from build123d import *

# Parameters (mm, degrees)
F1_DEPTH     = 20
F2_DEPTH     = 5
F3_R         = 6.25
F4_DEPTH     = 10
F5_R         = 1.4
F6_DEPTH     = 3.9098179487
F7_T1_DEPTH  = 47.5
F7_T3_DEPTH  = 32.5
F7_T5_DEPTH  = 20.5
F7_T7_DEPTH  = 35.5
F7_T9_DEPTH  = 10
F7_S13_W     = 5
F7_S13_H     = 5
F7_T14_DEPTH = 5
F7_S19_W     = 5
F7_S19_H     = 5
F7_T20_DEPTH = 5
F7_T27_DEPTH = 45
F7_T31_DEPTH = 33
F7_T38_DEPTH = 45
F7_T42_DEPTH = 33


# Not quite as in the source:
# - a fillet or chamfer that OpenCascade refuses, or shapes differently, is made with other operations: its cross-section is extruded or revolved along the edge and cut away or added


with BuildPart() as f1:
    # F0 (on Top) → F1 (new body)
    with BuildSketch(Plane.XY):
        Polygon((0, 10), (0, 0), (0, -10), (20, -10), (20, -18), (40, -18), (40, 10), align=None)
        Polygon((35.5, -12), (35.5, -17.5), (30, -17.5), (24.5, -17.5), (24.5, -12), align=None, mode=Mode.SUBTRACT)
    extrude(amount=F1_DEPTH)

    # F0 (on Top) → F2 (join)
    with BuildSketch(Plane.XY):
        Polygon((30, -17.5), (35.5, -17.5), (35.5, -12), (24.5, -12), (24.5, -17.5), align=None)
    extrude(amount=F2_DEPTH)

    # F3 (on face) → F4 (cut)
    with BuildSketch(Plane(origin=(0, 0, 0), x_dir=(0, -1, 0), z_dir=(-1, 0, 0))):
        with Locations((0, 10)):
            Circle(F3_R)
    extrude(amount=-F4_DEPTH, mode=Mode.SUBTRACT)

    # F5 (on face) → F6 (cut, through all)
    with BuildSketch(Plane(origin=(0, 10, 0), x_dir=(-1, 0, 0), z_dir=(0, 1, 0))):
        with Locations((-5, 10)):
            Circle(F5_R)
    extrude(amount=-F6_DEPTH, mode=Mode.SUBTRACT)

    # F7: fillet of radius 5 on 9 edges, made by hand

    # F7_s2 → F7_t1 (cut)
    with BuildSketch(Plane.YZ.offset(-12.5)):
        with BuildLine():
            ThreePointArc((10, 15), (8.5355339059, 18.5355339059), (5, 20))
            Line((5, 20), (10, 20))
            Line((10, 20), (10, 15))
        make_face()
        with BuildLine():
            ThreePointArc((10, 5), (8.5355339059, 1.4644660941), (5, 0))
            Line((5, 0), (10, 0))
            Line((10, 0), (10, 5))
        make_face()
    extrude(amount=F7_T1_DEPTH, mode=Mode.SUBTRACT)

    # F7_s4 → F7_t3 (cut)
    with BuildSketch(Plane.YZ.offset(-12.5)):
        with BuildLine():
            ThreePointArc((-5, 20), (-8.5355339059, 18.5355339059), (-10, 15))
            Line((-10, 15), (-10, 20))
            Line((-10, 20), (-5, 20))
        make_face()
        with BuildLine():
            ThreePointArc((-5, 0), (-8.5355339059, 1.4644660941), (-10, 5))
            Line((-10, 5), (-10, 0))
            Line((-10, 0), (-5, 0))
        make_face()
    extrude(amount=F7_T3_DEPTH, mode=Mode.SUBTRACT)

    # F7_s6 → F7_t5 (cut)
    with BuildSketch(Plane.XZ.offset(10)):
        with BuildLine():
            ThreePointArc((25, 20), (21.4644660941, 18.5355339059), (20, 15))
            Line((20, 15), (20, 20))
            Line((20, 20), (25, 20))
        make_face()
        with BuildLine():
            ThreePointArc((25, 0), (21.4644660941, 1.4644660941), (20, 5))
            Line((20, 5), (20, 0))
            Line((20, 0), (25, 0))
        make_face()
    extrude(amount=F7_T5_DEPTH, mode=Mode.SUBTRACT)

    # F7_s8 → F7_t7 (cut)
    with BuildSketch(Plane.XZ.offset(-5)):
        with BuildLine():
            ThreePointArc((35, 20), (38.5355339059, 18.5355339059), (40, 15))
            Line((40, 15), (40, 20))
            Line((40, 20), (35, 20))
        make_face()
        with BuildLine():
            ThreePointArc((35, 0), (38.5355339059, 1.4644660941), (40, 5))
            Line((40, 5), (40, 0))
            Line((40, 0), (35, 0))
        make_face()
    extrude(amount=F7_T7_DEPTH, mode=Mode.SUBTRACT)

    # F7_s10 → F7_t9 (cut)
    with BuildSketch(Plane.XY.offset(5)):
        with BuildLine():
            ThreePointArc((35, 10), (38.5355339059, 8.5355339059), (40, 5))
            Line((40, 5), (40, 10))
            Line((40, 10), (35, 10))
        make_face()
    extrude(amount=F7_T9_DEPTH, mode=Mode.SUBTRACT)


with BuildPart() as f7_tool12:
    # F7_s13 → F7_t14 (new body)
    with BuildSketch(Plane.XZ.offset(-5)):
        with Locations((37.5, 17.5)):
            Rectangle(F7_S13_W, F7_S13_H)
    extrude(amount=-F7_T14_DEPTH)

    # F7_s15 → F7_t16 (revolve, cut)
    with BuildSketch(Plane(origin=(35, 5, 15), x_dir=(-0.7071067812, 0, -0.7071067812), z_dir=(0.7071067812, 0, -0.7071067812))):
        with BuildLine():
            ThreePointArc((0, -5), (5, 0), (0, 5))
            Line((0, 5), (0, -5))
        make_face()
    revolve(axis=Axis((35, 5, 15), (0, 1, 0)), mode=Mode.SUBTRACT)


with BuildPart() as f1_1:
    add(f1.part)

    # F7_t11: cut F7_tool12
    add(f7_tool12.part, mode=Mode.SUBTRACT)


with BuildPart() as f7_tool18:
    # F7_s19 → F7_t20 (new body)
    with BuildSketch(Plane.XZ.offset(-5)):
        with Locations((37.5, 2.5)):
            Rectangle(F7_S19_W, F7_S19_H)
    extrude(amount=-F7_T20_DEPTH)

    # F7_s21 → F7_t22 (revolve, cut)
    with BuildSketch(Plane(origin=(35, 5, 5), x_dir=(-0.7071067812, 0, 0.7071067812), z_dir=(-0.7071067812, 0, -0.7071067812))):
        with BuildLine():
            ThreePointArc((0, -5), (5, 0), (0, 5))
            Line((0, 5), (0, -5))
        make_face()
    revolve(axis=Axis((35, 5, 5), (0, 1, 0)), mode=Mode.SUBTRACT)


with BuildPart() as f1_2:
    add(f1_1.part)

    # F7_t17: cut F7_tool18
    add(f7_tool18.part, mode=Mode.SUBTRACT)


with BuildPart() as f7_tool25:
    # F7_s26 → F7_t27 (new body)
    with BuildSketch(Plane.YZ.offset(-12.5)):
        with BuildLine():
            ThreePointArc((-5, 20), (-8.5355339059, 18.5355339059), (-10, 15))
            Line((-10, 15), (-10, 20))
            Line((-10, 20), (-5, 20))
        make_face()
    extrude(amount=F7_T27_DEPTH)

    split(bisect_by=Plane.YZ.offset(20), keep=Keep.TOP)


with BuildPart() as f7_tool29:
    # F7_s30 → F7_t31 (new body)
    with BuildSketch(Plane.XZ.offset(-2.5)):
        with BuildLine():
            ThreePointArc((25, 20), (21.4644660941, 18.5355339059), (20, 15))
            Line((20, 15), (20, 20))
            Line((20, 20), (25, 20))
        make_face()
    extrude(amount=F7_T31_DEPTH)

    split(bisect_by=Plane.XZ.offset(10), keep=Keep.BOTTOM)


with BuildPart() as f7_tool25_1:
    add(f7_tool25.part)

    # F7_t33: intersect F7_tool29
    add(f7_tool29.part, mode=Mode.INTERSECT)


with BuildPart() as f1_3:
    add(f1_2.part)

    # F7_t23: cut F7_tool25
    add(f7_tool25_1.part, mode=Mode.SUBTRACT)


with BuildPart() as f7_tool36:
    # F7_s37 → F7_t38 (new body)
    with BuildSketch(Plane.YZ.offset(-12.5)):
        with BuildLine():
            ThreePointArc((-5, 0), (-8.5355339059, 1.4644660941), (-10, 5))
            Line((-10, 5), (-10, 0))
            Line((-10, 0), (-5, 0))
        make_face()
    extrude(amount=F7_T38_DEPTH)

    split(bisect_by=Plane.YZ.offset(20), keep=Keep.TOP)


with BuildPart() as f7_tool40:
    # F7_s41 → F7_t42 (new body)
    with BuildSketch(Plane.XZ.offset(-2.5)):
        with BuildLine():
            ThreePointArc((25, 0), (21.4644660941, 1.4644660941), (20, 5))
            Line((20, 5), (20, 0))
            Line((20, 0), (25, 0))
        make_face()
    extrude(amount=F7_T42_DEPTH)

    split(bisect_by=Plane.XZ.offset(10), keep=Keep.BOTTOM)


with BuildPart() as f7_tool36_1:
    add(f7_tool36.part)

    # F7_t44: intersect F7_tool40
    add(f7_tool40.part, mode=Mode.INTERSECT)


with BuildPart() as f1_4:
    add(f1_3.part)

    # F7_t34: cut F7_tool36
    add(f7_tool36_1.part, mode=Mode.SUBTRACT)


solid = f1_4.part
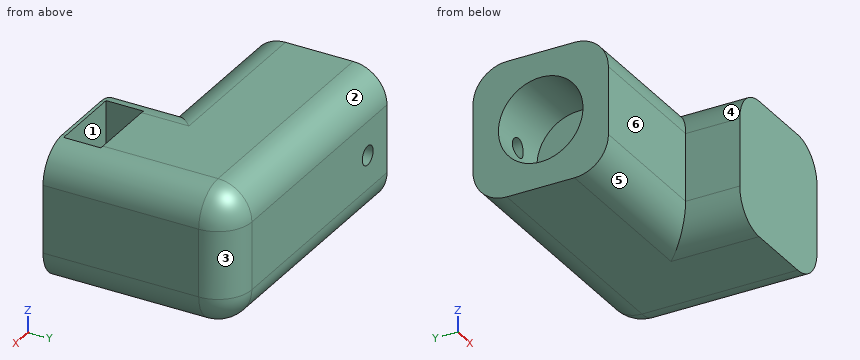
Source: CAD feature listing. Evaluate the final solid. Frame: model axes, mm. Face numbers are marked on the shaded views. A direction names the side the tool comes from. Round coordinates to 2 decimals unless told otherwise and drop trailing zeros. Write each loop counter-clockwise with the first axis right and the second up, starting at its lowest first coordinate (ties: lowest second). Pieces come first, ordered by that corner, then holes. Notation, with made-up numbers: M 37.25,-0.75 L 94.25,-0.75 A31 ccw 94.25,36.25 Z; hole C -18.5,-9 d3. An arc over 180 degrees is marked long. One line per item, written item: value. Start each with the question number.
Item 1: Pin query (flat end, axial travel): pin 1 (10 mm diameter, centred on x = 7, z = 5, fed in from -Y); pin 2 (6 mm diameter, centred on y = -3, z = 8.5, fed in from -X); pin 3 (2 mm diameter, centred on x = 17, z = 2.5, fed in from +Y); pin 4 (1.6 mm diameter, centred on y = -15, z = 13.5, fed in from -X). Return the tip coordinate at first contact, or that it passes through.
Item 2: Ray query, L1, parallel to Z at x = 2, y = 0; L2, parallel to Z at x = 7, y = 3.75; L3, parallel to Y at x = 30, z = 9.75. Return the intervals inside material, ascending. Write a range as from..to.
Item 3: Mould query, pull axis X, two halves, no side actions, for the marked faces 1, 2 and 3. Classes: pulls with the +X half, pulls with the -X half, needs draft (parallel to the pull), parting line crosses it, or undercut.
Item 4: Section query A-A (z = 10). Return the cut outline in (x, y), plus the area to 3 significant figures.
Item 5: Section query D-D (z = 12.75). Return the cut outline in (x, y).
Item 6: Section query C-C (y = -10.75). Return the cut outline in (x, z).
Item 7: Section query B-B (x = 30). Return the cut outline in (y, z).
Item 8: Set-up query: the marked faces 4, 5 and 6. Return all of +Z, -Z, +X, -X, +Y, -Y with unobstructed straight access to the full face (end or side cutting, diameter ignored); none if empty.
Result set:
1. pin 1: stops at y = -10
1. pin 2: stops at x = 0
1. pin 3: stops at y = 9.77
1. pin 4: stops at x = 20
2. L1: z = 0..3.75, 16.25..20
2. L2: z = 0..5, 15..20
2. L3: y = -18..-17.5, -12..10
3. face 1: undercut
3. face 2: needs draft
3. face 3: pulls with the +X half
4. outline: M 0,-10 L 20,-10 L 20,-18 L 40,-18 L 40,5 A5 ccw 35,10 L 6.4,10 L 6.4,6.25 L 10,6.25 L 10,-6.25 L 0,-6.25 Z; M 0,6.25 L 3.6,6.25 L 3.6,10 L 0,10 Z; hole M 24.5,-17.5 L 35.5,-17.5 L 35.5,-12 L 24.5,-12 Z
4. area: 759 mm²
5. outline: M 0,-10 L 20,-10 L 20,-18 L 40,-18 L 40,5 A5 ccw 35,10 L 0,10 L 0,5.61 L 10,5.61 L 10,-5.61 L 0,-5.61 Z; hole M 24.5,-17.5 L 35.5,-17.5 L 35.5,-12 L 24.5,-12 Z
6. outline: M 20,5 A5 ccw 25,0 L 35,0 A5 ccw 40,5 L 40,15 A5 ccw 35,20 L 25,20 A5 ccw 20,15 Z
7. outline: M -18,0 L 5,0 A5 ccw 10,5 L 10,15 A5 ccw 5,20 L -12,20 L -12,5 L -17.5,5 L -17.5,20 L -18,20 Z
8. face 4: +Z, -X, -Y
8. face 5: -Z, -X, -Y
8. face 6: +Z, -Z, -X, -Y
